Autodesk Fusion 360 part; units mm, degrees
sketch "Esquisse1" plane through (0, 0, 0) normal (0, 0, 1) x (1, 0, 0)
  line L0 (-40, 10) -> (40, 10)
  line L1 (40, 10) -> (40, -10)
  line L2 (40, -10) -> (-40, -10)
  line L3 (-40, -10) -> (-40, 10)
extrude "Extrusion1" add sketch "Esquisse1" along normal blind 10
sketch "Esquisse2" plane through (0, 0, 10) normal (0, 0, 1) x (-1, 0, 0)
  line L0 (40, 10) -> (-40, 10)
  line L1 (-40, 10) -> (-40, -10)
  line L2 (-40, -10) -> (40, -10)
  line L3 (40, -10) -> (40, 10)
  line L4 (15, -10) -> (-15, -10)
  line L5 (-15, -10) -> (-15, 10)
  line L6 (-15, 10) -> (15, 10)
  line L7 (15, 10) -> (15, -10)
  circle A0 centre (-31.183, 0) radius 1.625
  circle A1 centre (31.183, 0) radius 1.625
  dimension "d7" = 3.25
  dimension "d8" = 3.25
extrude "Extrusion2" cut sketch "Esquisse2" against normal blind 10 contours A1
extrude "Extrusion3" cut sketch "Esquisse2" against normal blind 10 contours A0
extrude "Extrusion4" add sketch "Esquisse2" along normal blind 30 contours L0 L2 L4 L5 L6 L7
sketch "Esquisse3" plane through (0, -10, 0) normal (0, -1, 0) x (1, 0, 0)
  line L0 (-40, 0) -> (40, 0)
  line L1 (40, 0) -> (40, 10)
  line L2 (40, 10) -> (15, 10)
  line L3 (15, 10) -> (15, 40)
  line L4 (15, 40) -> (-15, 40)
  line L5 (-15, 40) -> (-15, 10)
  line L6 (-15, 10) -> (-40, 10)
  line L7 (-40, 10) -> (-40, 0)
  circle A0 centre (0, 25) radius 6.5
  circle A1 centre (0, 25) radius 8
  dimension "d15" = 13
  dimension "d16" = 16
extrude "Extrusion5" cut sketch "Esquisse3" against normal blind 20 contours A0
extrude "Extrusion6" cut sketch "Esquisse3" against normal blind 5.1 contours A1
sketch "Esquisse4" plane through (0, 0, 40) normal (0, 0, 1) x (-1, 0, 0)
  line L0 (15, 10) -> (-15, 10)
  line L1 (-15, 10) -> (-15, -10)
  line L2 (-15, -10) -> (15, -10)
  line L3 (15, -10) -> (15, 10)
  line L4 (15, 10) -> (10, 10)
  line L5 (10, 10) -> (10, -5)
  line L6 (10, -5) -> (15, -5)
  line L7 (15, -5) -> (15, 10)
  line L8 (-15, 10) -> (-10, 10)
  line L9 (-10, 10) -> (-10, -5)
  line L10 (-10, -5) -> (-15, -5)
  line L11 (-15, -5) -> (-15, 10)
extrude "Extrusion7" add sketch "Esquisse4" along normal blind 10 contours L0 L3 L4 L5 L6 L7 | L0 L1 L8 L9 L10 L11
sketch "Esquisse5" plane through (0, 0, 50) normal (0, 0, 1) x (-1, 0, 0)
  line L0 (15, -5) -> (15, 10)
  line L1 (15, 10) -> (10, 10)
  line L2 (10, 10) -> (10, -5)
  line L3 (10, -5) -> (15, -5)
  line L4 (15, -5) -> (-15, -5)
  line L5 (-15, -5) -> (-15, 10)
  line L6 (-15, 10) -> (15, 10)
  line L7 (15, 10) -> (15, -5)
extrude "Extrusion8" add sketch "Esquisse5" along normal blind 5
Geometry check sheet. Reference: the model listing, model coordinates, mm. A direction names the side the tool comes from. Give positions to 0.01 mm unless a question says otherwise; leave off trailing zeros. Write each loop counter-clockwise with the first axis right and the second up, starting at its lowest first coordinate (ties: lowest second). Pieces come first, ordered by that corner, then holes.
1) Section check D-D, the plane y = -7. Record the boundary of the cut face in (x, z).
2) Section check B-B, the plane x = 0. Record the boundary of the cut face in (y, z), and give its area (3 significant figures).
3) Gauge pin test, flat ends, axial feed: pin 1 (10 mm diameter, centred on x = 28, y = 5.5, fed in from +Z); pin 2 (8 mm diameter, centred on y = -4.5, z = 47, fed in from +X); pin 3 (16.5 mm diameter, centred on x = -1, z = 49.5, fed in from +Y). Record the tip position at first contact, or that the pin passes through.
4) Access from +Z, -Z, +X, -X, +Y, -Y to the whole of each face (thin tool, end or side, straight path). Record for faces 1 (the flat face through (-1, 10, 15)), 2 (the cylindrical face through (-1.041, -7.486, 32.932)), 3 (the flat face through (-10, -3, 45)), 4 (the flat face through (0, 5, 51)), 5 (the flat face through (-28, 0, 10)).
5) Release check for a two-part mould opening along X. For faces 6 (the flat face through (15, 0, 32)), 7 (the cylindrical face through (32.806, -0.071, 5.07)), 8 (the flat face through (27, 0, 10)) record: pulls with the +X half, pulls with the -X half, needs draft (parallel to the pull), parting line crosses it, or undercut.
6) Section check A-A, the plane y = 0. Record the boundary of the cut face in (x, z).
7) Section check C-C, the plane z = 48. Record the boundary of the cut face in (x, y).
8) Material ranges on L1, parallel to X at y = -0.25, z = 7; L2, parallel to Z at x = 0.5, y = 0; L3, parallel to Z at x = 6, y = -4.25, recorded low to high.
Computed:
1. outline: (-40, 0) - (40, 0) - (40, 10) - (15, 10) - (15, 55) - (-15, 55) - (-15, 10) - (-40, 10) - close; hole (-10, 40) - (10, 40) - (10, 50) - (-10, 50) - close; hole circle Ø16 at (0, 25)
2. outline: (-10, 0) - (10, 0) - (10, 18.5) - (-4.9, 18.5) - (-4.9, 17) - (-10, 17) - close; (-10, 33) - (-4.9, 33) - (-4.9, 31.5) - (10, 31.5) - (10, 40) - (-10, 40) - close; (-10, 50) - (5, 50) - (5, 55) - (-10, 55) - close
2. area: 600 mm2
3. pin 1: stops at z = 10
3. pin 2: stops at x = 15
3. pin 3: stops at y = 5
4. face 1: +Z, -Z, +X, -X, +Y
4. face 2: -Y
4. face 3: +Y, -Y
4. face 4: +Z, +X, -X, +Y
4. face 5: +Z, -X, +Y, -Y
5. face 6: pulls with the +X half
5. face 7: undercut
5. face 8: needs draft
6. outline: (-40, 0) - (-32.81, 0) - (-32.81, 10) - (-40, 10) - close; (-29.56, 0) - (29.56, 0) - (29.56, 10) - (15, 10) - (15, 55) - (-15, 55) - (-15, 10) - (-29.56, 10) - close; (32.81, 0) - (40, 0) - (40, 10) - (32.81, 10) - close; hole (-10, 40) - (10, 40) - (10, 50) - (-10, 50) - close; hole circle Ø13 at (0, 25)
7. outline: (-15, -10) - (-10, -10) - (-10, 5) - (-15, 5) - close; (10, -10) - (15, -10) - (15, 5) - (10, 5) - close
8. L1: x = -40 to -32.79, -29.58 to 29.58, 32.79 to 40
8. L2: z = 0 to 18.52, 31.48 to 40, 50 to 55
8. L3: z = 0 to 22.5, 27.5 to 40, 50 to 55
